For this review, use the dimensioned drawing (mm, ordinates from the lowest corner) and the shaded views. Coordinates: 2 decimals unless noted, no trailing zeros. Order: outer loops, then holes, each group sorted by start corner. A loop starts at its lowest first (then second) coordinate and runs counter-clockwise, first axis right, second up. Notation, with made-up numbers: M 11.25,13 L 68.25,13 A7 cw 68.25,25 Z; hole C 24,-14.5 d6. An arc over 180 degrees is marked long. Use CSV: the item, a comma, the result in double quotes.
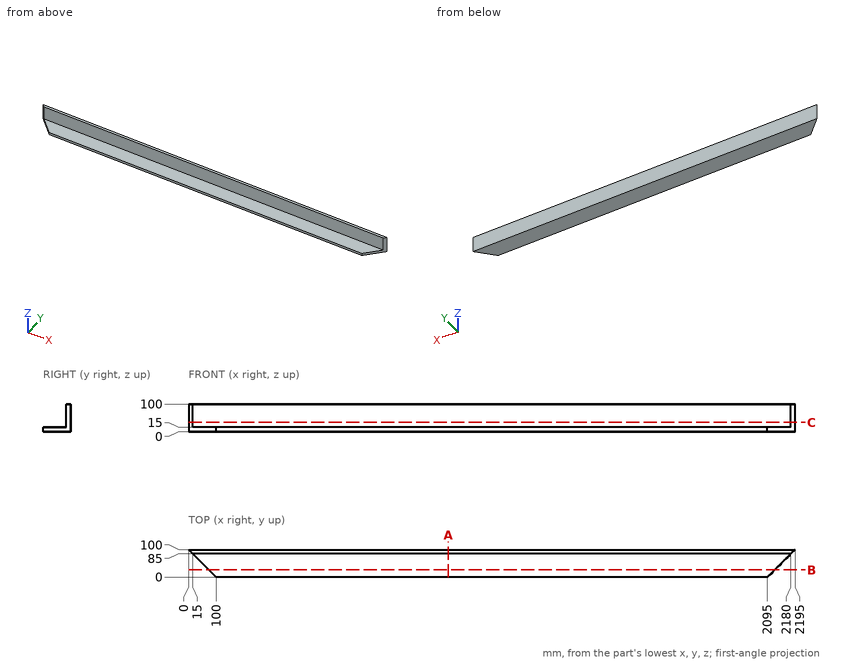
Item 1: Add section C-C on z = 33.5. State the section outline as (x, y) points, and give its area (3 significant figures).
Solutions:
outline,"M 0,100 L 15,85 L 2180,85 L 2195,100 Z"
area,"32,700 mm^2"
Item 2: To check wall thickness, follow line 1 along Z through (x, y) = (148, 6.5); line 2 along Y through (x, z) = (1265, 20.5); line 3 along X through (y, z) = (95, 69). State the ranges of each line that lie inside material, in increasing order. Write a range as [from, to].
Solutions:
line 1,"[0, 15]"
line 2,"[85, 100]"
line 3,"[5, 2190]"
Item 3: Add section A-A on x = 940.5. State the section outline as (y, z) points.
Solutions:
outline,"M 0,0 L 100,0 L 100,100 L 85,100 L 85,15 L 0,15 Z"
Item 4: Clearance check with flat-ended pins moving along their axes: pin 1 Ø12 at (x, y) = (1023, 29.5) entering from -Z; pin 2 Ø1.5 at (x, y) = (1038.5, 42.5) entering from +Z. State where each tip first meets the part, or that it passes through.
Solutions:
pin 1,"z = 0"
pin 2,"z = 15"
Item 5: Add section B-B on y = 27. State the section outline as (x, z) points.
Solutions:
outline,"M 73,0 L 2122,0 L 2122,15 L 73,15 Z"
